Answer from the drawing. Dimensions are ordinates in mm from the lowest x, y and z of the part. Round coordinates to 2 decimals unless told otherwise and drop trailing zeros. Loops run counter-clockwise (first coordinate to the right, second up) from the corner with the lowest first, then second, coordinate; pieces in that order, holes last.
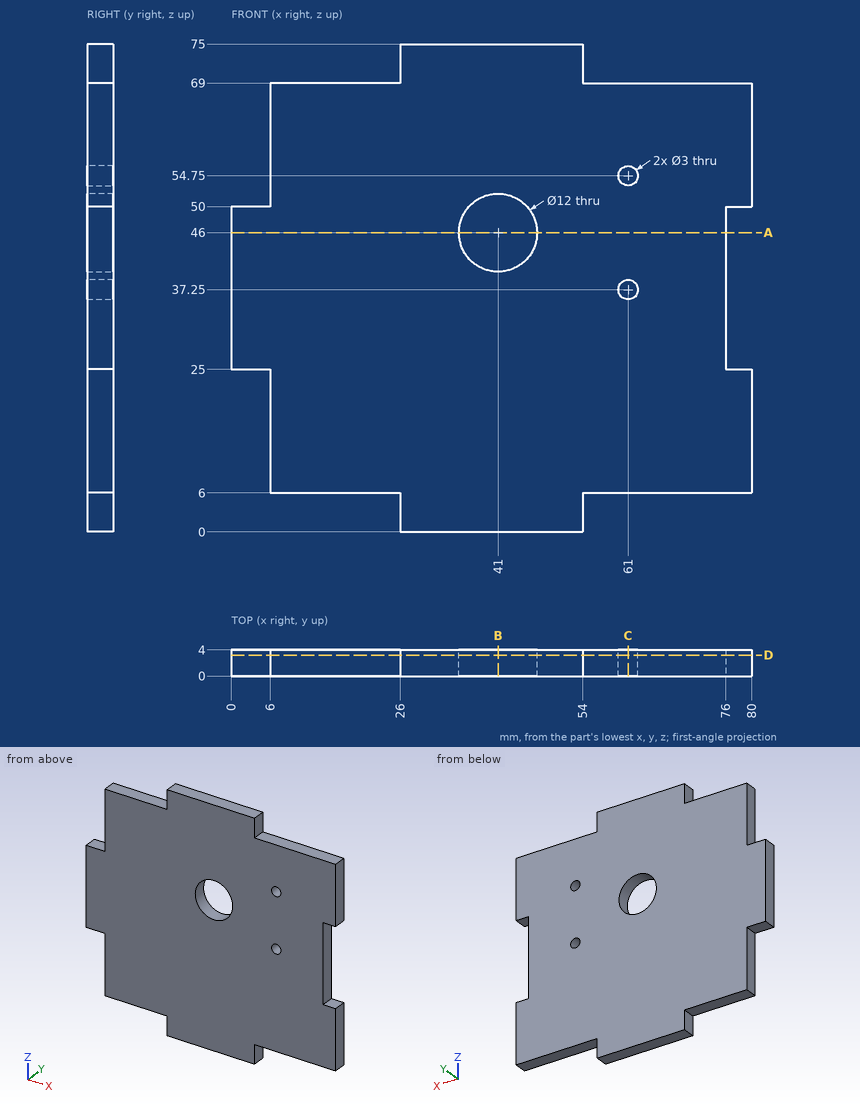
Item 1: Section D-D, the plane y = 3.2 is taken. Give the vertices of the cut face in (x, z), plus the area to 3 significant figures.
Item 2: Section B-B, the plane x = 41 is taken. Give the vertices of the cut face in (y, z).
Item 3: Straight lines are drawn through the part: line 1 (Z direction, x = 61, y = 2.55); line 2 (X direction, y = 2.1, z = 46); line 3 (Z direction, x = 62, y = 0.35). For each, find the intervals that lie inside material, in ascending order.
Item 4: Section C-C, the plane x = 61 is taken. Give the vertices of the cut face in (y, z).
Item 5: Each of these flat-tipped pins is pushed along its axis until it touches: P1, Ø1.2, axis at y = 3, z = 61.5, coming from the -X side; P2, Ø1.2, axis at y = 1.5, z = 71, coming from the -X side; P3, Ø2, axis at x = 77.5, y = 2.5, coming from the -Z side; P4, Ø1.8, axis at x = 61, z = 54.75, coming from the -Y side. Where does it stop, or does it pass through?
Item 6: Section A-A, the plane z = 46 is taken. Give the vertices of the cut face in (x, y).
Answer below:
1. outline: (0, 25) - (6, 25) - (6, 6) - (26, 6) - (26, 0) - (54, 0) - (54, 6) - (80, 6) - (80, 25) - (76, 25) - (76, 50) - (80, 50) - (80, 69) - (54, 69) - (54, 75) - (26, 75) - (26, 69) - (6, 69) - (6, 50) - (0, 50) - close; hole circle Ø12 at (41, 46); hole circle Ø3 at (61, 37.25); hole circle Ø3 at (61, 54.75)
1. area: 4,920 mm2
2. outline: (0, 0) - (4, 0) - (4, 40) - (0, 40) - close; (0, 52) - (4, 52) - (4, 75) - (0, 75) - close
3. line 1: z = 6 to 35.75, 38.75 to 53.25, 56.25 to 69
3. line 2: x = 0 to 35, 47 to 76
3. line 3: z = 6 to 36.13, 38.37 to 53.63, 55.87 to 69
4. outline: (0, 6) - (4, 6) - (4, 35.75) - (0, 35.75) - close; (0, 38.75) - (4, 38.75) - (4, 53.25) - (0, 53.25) - close; (0, 56.25) - (4, 56.25) - (4, 69) - (0, 69) - close
5. P1: stops at x = 6
5. P2: stops at x = 26
5. P3: stops at z = 6
5. P4: passes through
6. outline: (0, 0) - (35, 0) - (35, 4) - (0, 4) - close; (47, 0) - (76, 0) - (76, 4) - (47, 4) - close
